Could you check a few things on this model? Use its own coordinates, in mm. A direction names the side the tool comes from. Coordinates: 2 decimals unless noted, no trailing zeros. Loops run counter-clockwise (first coordinate to the right, second up) from the corner with the lowest first, then second, coordinate; pieces in that order, holes last. Notation, with made-up numbers: (2.5, -30.75) - (35.5, -30.75) arc R5 ccw to (35.5, -21.75) - close; hole circle Ø2 at (82, -39.75). An arc over 180 degrees is marked (long way). Use CSV: the item, a comma, the result in double quotes.
Autodesk Inventor part; units mm, degrees
ref_plane "РабПлоскость2" through (-265, -125, -86) normal (1, 0, 0) x (0, 1, 0)
ref_plane "YZ Plane" through (0, 0, 0) normal (1, 0, 0) x (0, 1, 0)
ref_plane "XZ Plane" through (0, 0, 0) normal (0, 1, 0) x (-1, 0, 0)
ref_plane "РабПлоскость1" through (0, 0, 0) normal (0, 0, 1) x (1, 0, 0)
sketch "Эскиз1" plane through (0, 0, 0) normal (0, 0, 1) x (1, 0, 0)
  line L0 (265, 175) -> (-265, 175)
  line L1 (-265, 175) -> (-265, -175)
  line L2 (-265, 125) -> (-245, 125)
  line L3 (-245, 125) -> (-245, 143)
  line L4 (-245, 143) -> (-230, 158)
  line L5 (-230, 158) -> (-149.3726, 158)
  line L6 (-149.3726, 158) -> (-149.3726, 178)
  point P0 (0, 0)
  point P1 (-149.3726, 175)
extrude "Выдавливание1" add sketch "Эскиз1" along normal blind 15.7
sketch "Эскиз2" plane through (-245, 125, 0) normal (1, 0, 0) x (0, 0, -1)
  line L0 (0, 0) -> (-15.7, 0)
  line L1 (-20, -4) -> (0, -38.641)
  line L2 (-20, -4) -> (-20, 0)
  line L3 (0, 50) -> (0, -300)
  line L4 (-20, 0) -> (-15.7574, 0)
  line L5 (-20, 0) -> (0, 0)
  line L6 (0, -38.641) -> (0, 0)
  point P0 (0, -125)
  point P1 (-1, -36.909)
  point P2 (-1, 0)
  point P3 (-1, 0)
ref_plane "РабПлоскость2" through (-265, -125, -86) normal (1, 0, 0) x (0, 1, 0)
extrude "Выдавливание2" add sketch "Эскиз2" against normal up to surface (20 mm away)
sketch "Эскиз3" plane through (-230, 158, 0) normal (0, -1, 0) x (1, 0, 0)
  line L0 (91.2262, -0.185) -> (79.9532, 15.7574)
  line L1 (80.6274, 0) -> (80.6274, 15.7)
  line L2 (0, 0) -> (80.6274, 0)
  line L3 (80.6274, 0) -> (91.2262, -0.185)
  point P0 (230, 0)
  point P1 (80.6274, 14.8038)
extrude "Выдавливание3" add sketch "Эскиз3" against normal blind 10.75
sketch "Эскиз4" plane through (0, 0, 0) normal (0, 0, -1) x (-1, 0, 0)
  line L0 (245, 143) -> (230, 158)
  line L1 (230, 158) -> (149.3726, 158)
  line L2 (245, 86.359) -> (245, 143)
  line L3 (149.3726, 158) -> (138.7738, 158)
  line L4 (148.7738, 143) -> (149.3726, 143)
  line L5 (149.3726, 143) -> (223.7868, 143)
  line L6 (223.7868, 143) -> (230, 136.7868)
  line L7 (230, 136.7868) -> (230, 96.359)
  line L8 (138.7738, 153) -> (138.7738, 158)
  line L9 (240, 86.359) -> (245, 86.359)
  line L10 (240, 86.359) -> (230, 96.359)
  line L11 (148.7738, 143) -> (138.7738, 153)
  point P0 (0, 0)
  point P1 (138.7738, 143)
  point P2 (230, 86.359)
  point P3 (245, 88.091)
  dimension "d6" = 15
  dimension "d7" = 10
  dimension "d8" = 10
  dimension "d9" = 10
  dimension "d10" = 10
extrude "Выдавливание4" add sketch "Эскиз4" against normal blind 1
chamfer "Фаска1" distance 14.5 angle 45 3 edges at (-237.5, 150.5, 1) (-184.8059, 158, 1) (-245, 115.5455, 1)
sketch "Эскиз5" plane through (-245, 86.359, 15.5) normal (-1, 0, 0) x (0, 0, 1)
  point P0 (-15.5, -86.359)
sketch "Эскиз6" plane through (-245, 86.359, 15.5) normal (-1, 0, 0) x (0, 0, 1)
  line L0 (-15.5, 0) -> (0, 0)
  line L1 (0, 26.8468) -> (-15.5, 0)
  line L2 (0, 26.8468) -> (0, 0)
  point P0 (-15.5, -86.359)
extrude "Выдавливание5" cut sketch "Эскиз6" against normal blind 19.5
sketch "Эскиз7" plane through (-149.3726, 158, 15.5) normal (0, 1, 0) x (1, 0, 0)
  line L0 (10.5987, 15.5) -> (10.5987, 0)
  line L1 (10.4679, 15.5) -> (10.5987, 15.5)
  line L2 (10.4679, 15.5) -> (0, 0.6962)
  line L3 (0, 0.6962) -> (0, 0)
  line L4 (0, 0) -> (10.5987, 0)
  point P0 (149.3726, 15.5)
extrude "Выдавливание6" cut sketch "Эскиз7" against normal blind 19.5
sketch "Эскиз8" plane through (0, 0, 15.7) normal (0, 0, 1) x (1, 0, 0)
  circle A0 centre (-164.3726, 165) radius 3.25
  circle A1 centre (-228.3726, 165) radius 3.25
  point P0 (0, 0)
extrude "Выдавливание7" cut sketch "Эскиз8" against normal blind 28.75
sketch "Эскиз9" plane through (-230, 158, 15.7) normal (0, -1, 0) x (1, 0, 0)
  line L0 (86.8003, -9.6259) -> (80.6274, -0.8962)
  line L1 (81.7345, -2.4619) -> (79.5689, 0.6008)
  line L2 (79.5689, 0.6008) -> (81.1742, 0.6008)
  line L3 (81.1742, 0.6008) -> (81.1742, -1.6694)
  point P0 (230, -15.7)
  point P1 (80.6274, -0.8962)
  point P2 (81.1742, -1.6694)
extrude "Выдавливание8" cut sketch "Эскиз9" along normal through all both and the other way through all
properties part number "Накладка_левая"
(1) Which directions (+Z, -Z, +X, -X, +Y, -Y) give clear straight access to the entire face, cutting with the end or side of a thin tool? Please do faces 5 (the face through (-149.373, 172, 7)), 6 (the face through (-221, 161, 15.7)), 7 (the face through (-186, 150.6, 8.1)).
Computed:
face 5,"+Z, -Z, +X, +Y"
face 6,"+Z, +X, -X, +Y"
face 7,"+Z, +X, -Y"
(2) Suppose I cut it at B-B (y = 141). Write out the boundary of the cut face in (x, z).
Computed:
outline,"(-265, 0) - (-225.79, 0) - (-225.79, 1) - (-226.49, 1) - (-240.17, 10.67) - (-245, 15.5) - (-245, 15.7) - (-265, 15.7) - close"
(3) Will these pins go through, and if not, where does the flat tip stop? pin 1 (7 mm diameter, centred on y = 171, z = 4, fed in from +X); pin 2 (8 mm diameter, centred on x = -177, z = 2.5, fed in from -Y); pin 3 (4 mm diameter, centred on x = -228.37, y = 165, fed in from +Z); pin 4 (10.5 mm diameter, centred on x = -164.37, y = 165, fed in from +Z).
Computed:
pin 1,"stops at x = -139.84"
pin 2,"stops at y = 143"
pin 3,"passes through"
pin 4,"stops at z = 15.7"
(4) Suppose I cut it at D-D (y = 170). Write out the boundary of the cut face in (x, z).
Computed:
outline,"(-265, 0) - (-149.37, 0) - (-149.37, 14.8) - (-150.01, 15.7) - (-265, 15.7) - close"
(5) Suppose I cut it at A-A (x = -159). Write out the boundary of the cut face in (y, z).
Computed:
outline,"(143, 0) - (175, 0) - (175, 15.7) - (158, 15.7) - (158, 15.5) - (143.5, 1) - (143, 1) - close"
(6) Suppose I cut it at C-C (x = -242.5). Write out the boundary of the cut face in (y, z).
Computed:
outline,"(86.36, 0) - (175, 0) - (175, 15.7) - (145.5, 15.7) - (145.5, 15.5) - (141.96, 13) - (108.88, 13) - close"
(7) Thinking about a two-plate mould opening in Y: for faces 1 (the face through (-233.96, 92.4, 1.04)), 2 (the face through (-237.6, 117.7, 8.1)), 3 (the face through (-206, 175, 8)), 4 (the face through (-166.768, 167.197, 7.96)), which applies, +Y half, -Y half, draft (parallel to the pull), parting line (faces both ways), or undercut?
Computed:
face 1,"-Y half"
face 2,"draft"
face 3,"+Y half"
face 4,"undercut"
(8) Please list where these lines run through material, in increasing order: line 1 (X direction, y = 165, z = 3.75); line 2 (X direction, y = 165, z = 10.5); line 3 (Y direction, x = -171, z = 0.5).
Computed:
line 1,"x = -265 to -231.62, -225.12 to -167.62, -161.12 to -141.56"
line 2,"x = -265 to -231.62, -225.12 to -167.62, -161.12 to -146.33"
line 3,"y = 143 to 175"
